```python
from build123d import *

# Parameters (mm, degrees)
F0_R     = 26.75
F0_R_2   = 3
F0_R_3   = 1.6
F0_R_4   = 1.85
F0_R_5   = 0.75
F1_DEPTH = 2


# Not quite as in the source:
# - a feature names something its author has since deleted; it is built from what else it names


with BuildPart() as f1:
    # F0 (on Top) → F1 (new body)
    with BuildSketch(Plane.XY):
        Circle(F0_R)
        with Locations((0, -20)):
            Circle(F0_R_2, mode=Mode.SUBTRACT)
        with Locations((-17, 0)):
            Circle(F0_R_3, mode=Mode.SUBTRACT)
        with BuildLine():
            Line((-8.081475452, 13.081475452), (13.081475452, 13.081475452))
            Line((13.081475452, 13.081475452), (13.081475452, -8.081475452))
            ThreePointArc((13.081475452, -8.081475452), (16.6170093579, -9.545941546), (18.081475452, -13.081475452))
            ThreePointArc((18.081475452, -13.081475452), (13.081475452, -18.081475452), (8.081475452, -13.081475452))
            Line((8.081475452, -13.081475452), (-8.081475452, -13.081475452))
            ThreePointArc((-8.081475452, -13.081475452), (-16.6170093579, -16.6170093579), (-13.081475452, -8.081475452))
            Line((-13.081475452, -8.081475452), (-13.081475452, 8.081475452))
            ThreePointArc((-13.081475452, 8.081475452), (-16.6170093579, 16.6170093579), (-8.081475452, 13.081475452))
        make_face(mode=Mode.SUBTRACT)
        with Locations((0, 20)):
            Circle(F0_R_2, mode=Mode.SUBTRACT)
        with Locations((17, 6.6)):
            Circle(F0_R_4, mode=Mode.SUBTRACT)
        with Locations((9.5, 23)):
            Circle(F0_R_5, mode=Mode.SUBTRACT)
        with BuildLine():
            Line((13.081475452, -8.081475452), (13.081475452, 13.081475452))
            Line((13.081475452, 13.081475452), (-8.081475452, 13.081475452))
            ThreePointArc((-8.081475452, 13.081475452), (-9.545941546, 9.545941546), (-13.081475452, 8.081475452))
            Line((-13.081475452, 8.081475452), (-13.081475452, -8.081475452))
            ThreePointArc((-13.081475452, -8.081475452), (-9.545941546, -9.545941546), (-8.081475452, -13.081475452))
            Line((-8.081475452, -13.081475452), (8.081475452, -13.081475452))
            ThreePointArc((8.081475452, -13.081475452), (9.545941546, -9.545941546), (13.081475452, -8.081475452))
        make_face()
        Circle(F0_R_3, mode=Mode.SUBTRACT)
    extrude(amount=F1_DEPTH)


solid = f1.part
```
The listing builds one solid part. Answer for the finished solid, in the listing's coordinates (mm). Coordinates: 2 decimals unless noted, no trailing zeros. Loops run counter-clockwise (first coordinate to the right, second up) from the corner with the lowest first, then second, coordinate; pieces in that order, holes last. Notation, with made-up numbers: (84, 32.5) -> (109, 32.5) arc R12 ccw to (109, 39.5) -> close; hole circle Ø11 at (86.5, 7.25). An arc over 180 degrees is marked (long way). Use one line per item in the form item = value. Start each with the question number.
Item 1: The part is cut by section B-B on x = 0. Determine the outline of the cut face in (y, z).
Item 2: The part is cut by section C-C on z = 0.45. Count the separate pieces of the cut face and the enclosed holes in it, then the cut area to 3 significant figures.
Item 3: The part is cut by section D-D on y = 0. Determine the outline of the cut face in (x, z), then the cut area to 3 significant figures.
Item 4: Flat-ended cylindrical pins translate along their axes: pin 1 Ø3 at (x, y) = (17, 6.6) entering from +Z; pin 2 Ø1 at (x, z) = (-6.5, 0.5) entering from -Y; pin 3 Ø1 at (x, z) = (-4, 1.5) entering from -Y. Find the tip coordinate at first contact, or state that the pin passes through.
Item 5: The part is cut by section A-A on y = 6.6. Determine the outline of the cut face in (x, z).
Item 6: Consider L1, parallel to Y at x = 2, z = 0.2; L2, parallel to Y at x = 16.5, z = 1.9; L3, parallel to X at y = 11.5, z = 0.85. Determine where each line is inside the solid, lowest interval first. Write a range as [from, to].
Answer key:
q1.outline = (-26.75, 0) -> (-23, 0) -> (-23, 2) -> (-26.75, 2) -> close; (-17, 0) -> (-1.6, 0) -> (-1.6, 2) -> (-17, 2) -> close; (1.6, 0) -> (17, 0) -> (17, 2) -> (1.6, 2) -> close; (23, 0) -> (26.75, 0) -> (26.75, 2) -> (23, 2) -> close
q2.separate_pieces = 1
q2.enclosed_holes = 9
q2.area = 1,930 mm2
q3.outline = (-26.75, 0) -> (-18.6, 0) -> (-18.6, 2) -> (-26.75, 2) -> close; (-15.4, 0) -> (-1.6, 0) -> (-1.6, 2) -> (-15.4, 2) -> close; (1.6, 0) -> (26.75, 0) -> (26.75, 2) -> (1.6, 2) -> close
q3.area = 94.2 mm2
q4.pin_1 = through
q4.pin_2 = -26.07
q4.pin_3 = -26.52
q5.outline = (-25.92, 0) -> (15.15, 0) -> (15.15, 2) -> (-25.92, 2) -> close; (18.85, 0) -> (25.92, 0) -> (25.92, 2) -> (18.85, 2) -> close
q6.L1 = [-26.68, -22.24], [-17.76, 17.76], [22.24, 26.68]
q6.L2 = [-21.05, -16.73], [-9.43, 4.82], [8.38, 21.05]
q6.L3 = [-24.15, -17.82], [-8.34, 24.15]
